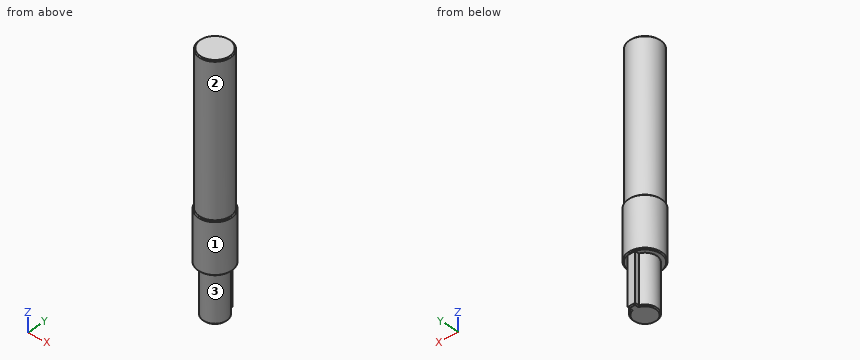
from build123d import *

# Parameters (mm, degrees)
SKETCH2_R           = 6
BOSS_EXTRUDE1_DEPTH = 25.4
BOSS_EXTRUDE2_START = 25
BOSS_EXTRUDE2_DEPTH = 25
SKETCH4_R           = 8.5
BOSS_EXTRUDE3_DEPTH = 26
SKETCH6_R           = 7.9375
BOSS_EXTRUDE4_DEPTH = 75.6
CHAMFER1_SIZE       = 0.5


with BuildPart() as part:
    # Sketch2 → Boss-Extrude1 (new body)
    with BuildSketch(Plane.XY):
        Circle(SKETCH2_R)
    extrude(amount=BOSS_EXTRUDE1_DEPTH)

    # Sketch3 → Boss-Extrude2 (add)
    with BuildSketch(Plane(origin=(0, 0, 0), x_dir=(-1, 0, 0), z_dir=(0, 0, -1)).offset(BOSS_EXTRUDE2_START)):
        with BuildLine():
            Line((-1.95, 5.674284096), (-1.95, 7.674284096))
            Line((-1.95, 7.674284096), (1.95, 7.674284096))
            Line((1.95, 7.674284096), (1.95, 5.674284096))
            ThreePointArc((1.95, 5.674284096), (0, -6), (-1.95, 5.674284096))
        make_face()
    extrude(amount=-BOSS_EXTRUDE2_DEPTH)

    # Sketch4 → Boss-Extrude3 (add)
    with BuildSketch(Plane.XY):
        with Locations(Location((0, 0, 0), (0, 0, 180))):
            Circle(SKETCH4_R)
    extrude(amount=BOSS_EXTRUDE3_DEPTH)

    # Sketch6 → Boss-Extrude4 (add)
    with BuildSketch(Plane.XY.offset(26)):
        Circle(SKETCH6_R)
    extrude(amount=BOSS_EXTRUDE4_DEPTH)

    # Chamfer1
    chamfer1_edges = [part.edges().sort_by_distance(p)[0] for p in [
        (8.5, 0, 0),
        (8.5, 0, 26),
        (-7.9375, 0, 101.6),
        (0, -6, -25),
        (-1.95, 6.674284096, -25),
        (0, 7.674284096, -25),
        (1.95, 6.674284096, -25),
    ]]
    chamfer(chamfer1_edges, length=CHAMFER1_SIZE)


solid = part.part
Work out the finished part from the listing and answer in its coordinate system (mm). Face numbers are marked on the shaded views. A direction names the side the tool comes from. Give positions to 0.01 mm unless a question says otherwise; leave off trailing zeros. Write each loop counter-clockwise with the first axis right and the second up, starting at its lowest first coordinate (ties: lowest second). Pieces come first, ordered by that corner, then holes. Notation, with made-up numbers: M -21.5,16 L -7.5,16 A32 cw -7.5,44 Z; hole C 57.25,-33.75 d8. An arc over 180 degrees is marked long. Answer as CSV lines item,"result".
Q1. A cutting plane is placed at C-C on z = 45. Write down the section's boundary in (x, y) (1 decimal).
A:
outline,"C 0,0 d15.9"
Q2. Find the intervals of material crossed by probe 1 along Z at (x, y) = (6.25, -3.5); probe 2 along Y at (x, z) = (-0.5, 3.5); probe 3 along X at (y, z) = (0.5, 45), in increasing order. Write a range as [from, to].
A:
probe 1,"z = [0, 101.6]"
probe 2,"y = [-8.49, 8.49]"
probe 3,"x = [-7.92, 7.92]"
Q3. A cutting plane is placed at B-B on y = 0. Write down the section's boundary in (x, z).
A:
outline,"M -8.5,0.5 L -8,0 L -6,0 L -6,-24.5 L -5.5,-25 L 5.5,-25 L 6,-24.5 L 6,0 L 8,0 L 8.5,0.5 L 8.5,25.5 L 8,26 L 7.94,26 L 7.94,101.1 L 7.44,101.6 L -7.44,101.6 L -7.94,101.1 L -7.94,26 L -8,26 L -8.5,25.5 Z"
Q4. Given P1, Ø2, axis at y = 7, z = -9.5, coming from the +X side; P2, Ø1.5, axis at x = 1.5, z = 81.5, coming from the +Y side; P3, Ø1.5, axis at x = -1.5, z = 36, coming from the -Y side, each flat-ended and moving along its own axis, determine where each tip first touches the part or whether it passes through.
A:
P1,"stops at x = 1.95"
P2,"stops at y = 7.9"
P3,"stops at y = -7.9"
Q5. A cutting plane is placed at D-D on z = -5. Write down the section's boundary in (x, y), plus the area to 3 significant figures.
A:
outline,"M -1.95,5.67 A6 ccw long 1.95,5.67 L 1.95,7.67 L -1.95,7.67 Z"
area,"120 mm²"
Q6. A cutting plane is placed at A-A on x = 0. Write down the section's boundary in (y, z).
A:
outline,"M -8.5,0.5 L -8,0 L -6,0 L -6,-24.5 L -5.5,-25 L 7.17,-25 L 7.67,-24.5 L 7.67,0 L 8,0 L 8.5,0.5 L 8.5,25.5 L 8,26 L 7.94,26 L 7.94,101.1 L 7.44,101.6 L -7.44,101.6 L -7.94,101.1 L -7.94,26 L -8,26 L -8.5,25.5 Z"
Q7. A tool of negligible diameter and unlimited length cuts with its end or side. For the marked faces 1, 2 and 3, from which of +Z, -Z, +X, -X, +Y, -Y can it reach the whole face along a straight path? Write none if from no direction.
A:
face 1,"+Z, -Z"
face 2,"+Z"
face 3,"-Z"
